Solid Edge part; units mm, degrees
sketch "Sketch1" plane through (0, 0, 0) normal (0, -1, 0) x (1, 0, 0)
  circle A0 centre (0, 0) radius 1.5875
extrude "Protrusion1" add sketch "Sketch1" along normal blind 9.525
sketch "Sketch2" plane through (0, -9.525, 0) normal (0, -1, 0) x (1, 0, 0)
  circle A0 centre (0, 0) radius 3.1115
extrude "ExtrudedProtrusion_2" add sketch "Sketch2" along normal blind 2.2606
fillet "Round_1" radius 1.27 1 edges at (-3.1115, -11.7856, 0)
cosmetic_thread "Thread1"
properties part number "91772A133"
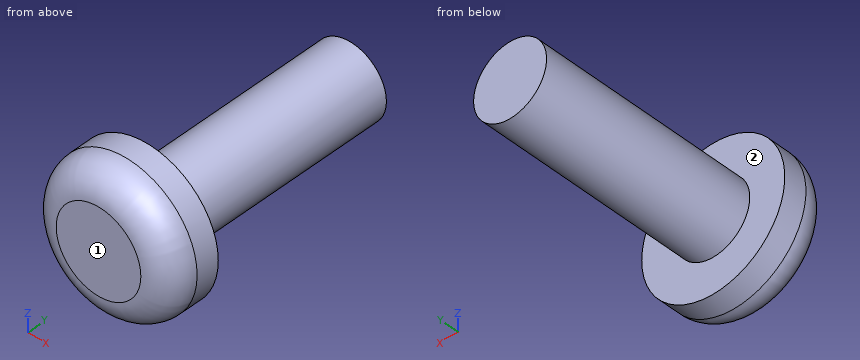
Here's how the part is built. I have some questions about the finished solid (model axes, mm). Face numbers are marked on the shaded views. A direction names the side the tool comes from. Coordinates: 2 decimals unless noted, no trailing zeros. Order: outer loops, then holes, each group sorted by start corner. A loop starts at its lowest first (then second) coordinate and runs counter-clockwise, first axis right, second up. Notation, with made-up numbers: (36, 78.25) - (68, 78.25) arc R10 cw to (68, 84.25) - close; hole circle Ø3 at (61, 88). An arc over 180 degrees is marked (long way). One line per question, with ' | ' between items.
(1) Suppose I cut it at A-A on x = 0. List the corners of the cut face in (y, z) for me (1 decimal), and give its area (3 significant figures).
Report:
outline: (-11.8, -1.8) arc R1.3 ccw to (-10.5, -3.1) - (-9.5, -3.1) - (-9.5, -1.6) - (0, -1.6) - (0, 1.6) - (-9.5, 1.6) - (-9.5, 3.1) - (-10.5, 3.1) arc R1.3 ccw to (-11.8, 1.8) - close | area: 43.6 mm2
(2) Suppose I cut it at B-B on z = 0. List the corners of the cut face in (x, y) for me (1 decimal), and give its area (3 significant figures).
Report:
outline: (-3.1, -10.5) arc R1.3 ccw to (-1.8, -11.8) - (1.8, -11.8) arc R1.3 ccw to (3.1, -10.5) - (3.1, -9.5) - (1.6, -9.5) - (1.6, 0) - (-1.6, 0) - (-1.6, -9.5) - (-3.1, -9.5) - close | area: 43.6 mm2
(3) Suppose I cut it at D-D on y = -9.75. List the corners of the cut face in (x, z) for me.
Report:
outline: circle Ø6.22 at (0, 0)
(4) Suppose I cut it at C-C on y = -5.25. List the corners of the cut face in (x, z) for me (1 decimal).
Report:
outline: circle Ø3.2 at (0, 0)
(5) If I drill on L1, parallel to Z at x = 0, y = -6.5; L2, parallel to Z at x = 1, y = -5.5; L3, parallel to Y at x = 0, z = -2 (3 decimals), over which ranges is the centre line in solid material (lowest first)?
Report:
L1: z = -1.59 to 1.59 | L2: z = -1.23 to 1.23 | L3: y = -11.776 to -9.525
(6) For the marked faces 1 and 2, which set-ups out of +Z, -Z, +X, -X, +Y, -Y let a thin tool reach every point of the face, with its end or its side?
Report:
face 1: +Z, -Z, +X, -X, -Y | face 2: +Y
(7) Will these pins go through, and if not, where does the flat tip stop? pin 1 (2 mm diameter, centred on x = -1.5, y = -4, fed in from -Z); pin 2 (2 mm diameter, centred on x = -0.5, y = -6, fed in from -Z).
Report:
pin 1: stops at z = -1.51 | pin 2: stops at z = -1.59
